Work out the finished part from the listing and answer in its coordinate system (mm). Face numbers are marked on the shaded views. A direction names the side the tool comes from. Give positions to 0.01 mm unless a question says otherwise; leave off trailing zeros. Order: outer loops, then holes, each group sorted by start corner. A loop starts at its lowest first (then second) coordinate and runs counter-clockwise, first axis right, second up.
```python
from build123d import *

# Parameters (mm, degrees)
BOSS_EXTRUDE1_DEPTH       = 28.575
SKETCH2_R                 = 17.4625
CUT_EXTRUDE1_DEPTH        = 26.19375
SKETCH3_R                 = 5
CUT_EXTRUDE2_DEPTH        = 39.404706031
F_8_32_TAPPED_HOLE1_D     = 3.4544
F_8_32_TAPPED_HOLE1_DEPTH = 5.588
F_8_32_TAPPED_HOLE1_TIP   = 1.037806461
SKETCH6_W                 = 5.08
SKETCH6_H                 = 5.08
BOSS_EXTRUDE2_DEPTH       = 3.175
FILLET1_R                 = 1.5875
CUT_EXTRUDE3_REACH        = 56.533
CUT_EXTRUDE3_END_RADIUS   = 17.4625
SKETCH7_R                 = 7.9375


with BuildPart() as part:
    # Sketch1 → Boss-Extrude1 (new body)
    with BuildSketch(Plane(origin=(0, 0, 0), x_dir=(0, 0, -1), z_dir=(1, 0, 0))):
        with BuildLine():
            Line((-19.05, 0), (-19.05, 20.6375))
            Line((-19.05, 20.6375), (19.05, 20.6375))
            Line((19.05, 20.6375), (19.05, 0))
            ThreePointArc((19.05, 0), (0, -19.05), (-19.05, 0))
        make_face()
    extrude(amount=BOSS_EXTRUDE1_DEPTH)

    # Sketch2 → Cut-Extrude1 (cut)
    with BuildSketch(Plane.ZY):
        Circle(SKETCH2_R)
    extrude(amount=-CUT_EXTRUDE1_DEPTH, mode=Mode.SUBTRACT)

    # Sketch3 → Cut-Extrude2 (cut, through all)
    with BuildSketch(Plane.ZY.offset(-26.19375)):
        Circle(SKETCH3_R)
    extrude(amount=-CUT_EXTRUDE2_DEPTH, mode=Mode.SUBTRACT)

    # #8-32 Tapped Hole1
    with Locations(Plane(origin=(0, 20.6375, 0), x_dir=(-1, 0, 0), z_dir=(0, 1, 0))):
        with Locations((-8.255, 12.7), (-8.255, -12.7), (-20.955, -12.7), (-20.955, 12.7), (-34.258152115, 14.428229267)):
            Hole(F_8_32_TAPPED_HOLE1_D / 2, depth=F_8_32_TAPPED_HOLE1_DEPTH)
            with Locations((0, 0, -(F_8_32_TAPPED_HOLE1_DEPTH + F_8_32_TAPPED_HOLE1_TIP / 2))):  # 118° drill point
                Cone(0, F_8_32_TAPPED_HOLE1_D / 2, F_8_32_TAPPED_HOLE1_TIP, mode=Mode.SUBTRACT)

    # Sketch6 → Boss-Extrude2 (add)
    with BuildSketch(Plane.ZY):
        with Locations((-21.59, 5.3975)):
            Rectangle(SKETCH6_W, SKETCH6_H)
    boss_extrude2 = extrude(amount=-BOSS_EXTRUDE2_DEPTH)

    # Mirror1: Boss-Extrude2 across plane
    add(boss_extrude2.mirror(Plane.XY))

    # Fillet1
    fillet1_edges = [part.edges().sort_by_distance(p)[0] for p in [
        (1.5875, 7.9375, -19.05),
        (1.5875, 2.8575, -19.05),
        (1.5875, 2.8575, -24.13),
        (1.5875, 7.9375, -24.13),
        (1.5875, 2.8575, 19.05),
        (1.5875, 7.9375, 19.05),
        (1.5875, 7.9375, 24.13),
        (1.5875, 2.8575, 24.13),
    ]]
    fillet(fillet1_edges, radius=FILLET1_R)

    # Cut-Extrude3: up to this cylinder (the profile starts outside it)
    cut_extrude3_end = Plane(origin=(14.2875, 0, 0), z_dir=(-1, 0, 0)) * Cylinder(CUT_EXTRUDE3_END_RADIUS, 148.991, mode=Mode.PRIVATE)
    # Sketch7 → Cut-Extrude3 (cut, up to the surface)
    with BuildSketch(Plane(origin=(0, 20.6375, 0), x_dir=(1, 0, 0), z_dir=(0, 1, 0)), mode=Mode.PRIVATE) as cut_extrude3_sk1:
        with Locations(Location((14.2875, 0, 0), (0, 0, 270))):
            Circle(SKETCH7_R)
    cut_extrude3_tool1 = extrude(cut_extrude3_sk1.sketch, amount=-CUT_EXTRUDE3_REACH, mode=Mode.PRIVATE) - cut_extrude3_end
    add(cut_extrude3_tool1.solids().sort_by_distance((14.2875, 20.6375, 0))[0], mode=Mode.SUBTRACT)


solid = part.part
```
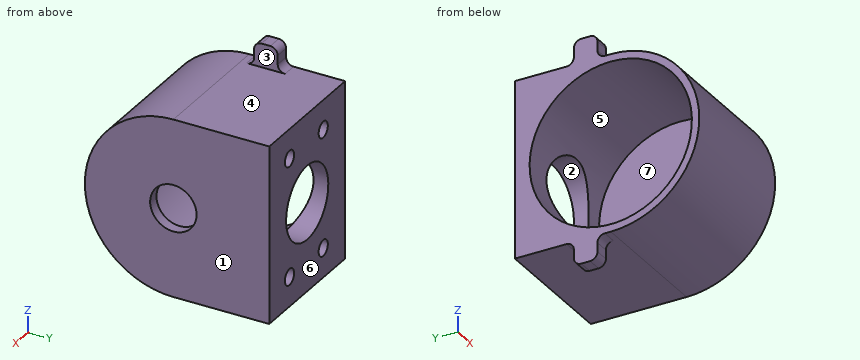
1. Given P1, Ø0.6, axis at x = 1, z = -22, coming from the -Y side; P2, Ø2.5, axis at y = 6, z = -21, coming from the +X side (3 decimals); P3, Ø5, axis at y = 11.5, z = 9.5, coming from the -X side, each flat-ended and moving along its own axis, determine where each tip first touches the part or whether it passes through.
Findings below:
P1: stops at y = 2.86
P2: stops at x = 3.175
P3: stops at x = 26.19
2. The mould has two halves that part along Y. Classify the marked faces 4, 5, 6 and 7: pulls with the +Y half, pulls with the -Y half, needs draft (parallel to the pull), parting line crosses it, or undercut.
Findings below:
face 4: needs draft
face 5: undercut
face 6: pulls with the +Y half
face 7: undercut
3. The part is cut by section D-D (z = 20). Write down the section's boundary in (x, y) (3 decimals).
Findings below:
outline: (0, 2.724) - (3.175, 2.724) - (3.175, 8.071) - (0, 8.071) - close
4. The part is cut by section A-A (z = 0). State how many separate pieces and enclosed holes the cut face has, then the cut area to 3 significant figures.
Findings below:
separate pieces: 3
enclosed holes: 0
area: 145 mm2
5. Which of the six approach directions +Z, -Z, +X, -X, +Y, -Y give full straight-line access (tool end or side, diameter ignored) to the marked faces 1, 2 and 3?
Findings below:
face 1: +Z, -Z, +X, +Y, -Y
face 2: +Y
face 3: +Z, +X, +Y, -Y
6. Straight lines are drawn through the part: probe 1 along X at (y, z) = (6, -8) (3 decimals); probe 2 along Y at (x, z) = (19, 8.5); probe 3 along Z at (x, y) = (6, 16). For each, find the intervals that lie inside material, in ascending order.
Findings below:
probe 1: x = 26.194 to 28.575
probe 2: y = -17.05 to -15.25, 15.25 to 20.64
probe 3: z = -19.05 to -7, 7 to 19.05
7. The part is cut by section B-B (y = -7). Write down the section's boundary in (x, z) (3 decimals).
Findings below:
outline: (0, -17.717) - (28.575, -17.717) - (28.575, 17.717) - (0, 17.717) - (0, 15.998) - (26.194, 15.998) - (26.194, -15.998) - (0, -15.998) - close
